The listing builds one solid part. Answer for the finished solid, in the listing's coordinates (mm). A direction names the side the tool comes from. Give positions to 0.01 mm unless a question says otherwise; leave off trailing zeros. Order: outer loops, then holes, each group sorted by start corner. A loop starts at its lowest first (then second) coordinate and runs counter-clockwise, first axis right, second up. Notation, with made-up numbers: M -33,9 L 16,9 A20 cw 16,22 Z; hole C 41,-13.5 d7. An arc over 180 degrees is marked long. Answer as a JSON object with one key per item and string values. Group by question number.
```python
from build123d import *

# Parameters (mm, degrees)
SKETCH1_R                          = 38.1
BOSS_EXTRUDE1_DEPTH                = 6.35
SKETCH2_R                          = 25.273
BOSS_EXTRUDE2_DEPTH                = 6.35
F_11_0_191_DIAMETER_HOLE1_D        = 4.8514
CIRPATTERN1_COUNT                  = 6
F_9_16_18_TAPPED_HOLE1_D           = 13.09624
F_9_16_18_TAPPED_HOLE1_CSINK_D     = 16.51
F_9_16_18_TAPPED_HOLE1_CSINK_ANGLE = 90
F_0_257_DIAMETER_HOLE1_D           = 6.5278


with BuildPart() as part:
    # Sketch1 → Boss-Extrude1 (new body)
    with BuildSketch(Plane(origin=(0, 0, 0), x_dir=(1, 0, 0), z_dir=(0, 1, 0))):
        with Locations(Location((0, 0, 0), (0, 0, 270))):
            Circle(SKETCH1_R)
    extrude(amount=BOSS_EXTRUDE1_DEPTH)

    # Sketch2 → Boss-Extrude2 (add)
    with BuildSketch(Plane(origin=(0, 0, 0), x_dir=(-1, 0, 0), z_dir=(0, -1, 0))):
        with Locations(Location((0, 0, 0), (0, 0, 270))):
            Circle(SKETCH2_R)
    extrude(amount=BOSS_EXTRUDE2_DEPTH)

    # #11 (0.191) Diameter Hole1 (through all)
    with Locations(Plane(origin=(0, 6.35, 0), x_dir=(1, 0, 0), z_dir=(0, 1, 0))):
        with Locations((0, 34.036)):
            f_11_0_191_diameter_hole1 = Hole(F_11_0_191_DIAMETER_HOLE1_D / 2)

    # CirPattern1: #11 (0.191) Diameter Hole1 ×6 about axis
    cirpattern1_axis = Axis((0, 0, 0), (0, 1, 0))
    for i in range(1, CIRPATTERN1_COUNT):
        add(f_11_0_191_diameter_hole1.rotate(cirpattern1_axis, i * 360 / CIRPATTERN1_COUNT), mode=Mode.SUBTRACT)

    # 9/16-18 Tapped Hole1 (through all)
    with Locations(Plane(origin=(0, 6.35, 0), x_dir=(1, 0, 0), z_dir=(0, 1, 0))):
        with Locations((0, 0)):
            CounterSinkHole(F_9_16_18_TAPPED_HOLE1_D / 2, F_9_16_18_TAPPED_HOLE1_CSINK_D / 2, counter_sink_angle=F_9_16_18_TAPPED_HOLE1_CSINK_ANGLE)

    # F (0.257) Diameter Hole1 (through all)
    with Locations(Plane(origin=(0, 6.35, 0), x_dir=(1, 0, 0), z_dir=(0, 1, 0))):
        with Locations((20.066, 0)):
            Hole(F_0_257_DIAMETER_HOLE1_D / 2)


solid = part.part
```
Item 1: Section C-C (y = 2.25) is taken. Count the separate pieces of the cut face and the enclosed holes in it, and give its area (3 significant figures).
Item 2: Section A-A (z = 0) is taken. Determine the outline of the cut face in (x, y) (3 decimals), and give its area (3 significant figures).
Item 3: Determine the mould class of faces 3 (the cylindrical face through (-27.235, 3.131, -17.947)), 4 (the cylindrical face through (9.68, -3.131, 23.346)), 5 (the flat face through (5, -6.35, 5)) for opening direction X: released by +X, released by -X, zero draft, split by the parting line, or undercut.
Item 4: Section D-D (x = -13) is taken. Determine the outline of the cut face in (y, z).
Item 5: Flat-ended cylindrical pins translate along their axes: P1, Ø3, axis at y = 3, z = 22.5, coming from the +X side; P2, Ø6.5, axis at x = -29.48, z = -17.02, coming from the -Y side; P3, Ø4, axis at y = -0.5, z = 16.5, coming from the +X side. Find the tip coordinate at first contact, or state that the pin passes through.
Item 6: A tool of negligible diameter and unlimited length cuts with its end or side. For faces 1 (the flat face through (-25, 0, 8)), 2 (the cylindrical face through (0.32, 3.13, -36.44)), from which of +Z, -Z, +X, -X, +Y, -Y can it reach the whole face along a straight path? Write none if from no direction.
Item 7: Consider probe 1 along Z at (x, y) = (-0.5, -4.5); probe 2 along X at (y, z) = (-2.5, -2); probe 3 along Y at (x, z) = (-14, 22.5). Determine where each line is inside the solid, lowest interval first. Write a range as from..to.
Item 8: Section B-B (x = 19.5) is taken. Determine the outline of the cut face in (y, z).
Values found:
{
 "1": {"separate pieces": "1", "enclosed holes": "8", "area": "4,280 mm^2"},
 "2": {"outline": "M -38.1,0 L -25.273,0 L -25.273,-6.35 L -6.548,-6.35 L -6.548,4.643 L -8.255,6.35 L -38.1,6.35 Z; M 6.548,-6.35 L 16.802,-6.35 L 16.802,6.35 L 8.255,6.35 L 6.548,4.643 Z; M 23.33,-6.35 L 25.273,-6.35 L 25.273,0 L 38.1,0 L 38.1,6.35 L 23.33,6.35 Z", "area": "553 mm^2"},
 "3": {"face 3": "undercut", "face 4": "split by the parting line", "face 5": "zero draft"},
 "4": {"outline": "M -6.35,-21.67 L 0,-21.67 L 0,-35.81 L 6.35,-35.81 L 6.35,35.81 L 0,35.81 L 0,21.67 L -6.35,21.67 Z"},
 "5": {"P1": "stops at x = 31.79", "P2": "stops at y = 0", "P3": "stops at x = 35.21"},
 "6": {"face 1": "-Y", "face 2": "+Y, -Y"},
 "7": {"probe 1": "z = -25.27..-6.53, 6.53..25.27", "probe 2": "x = -25.19..-6.24, 6.24..17.49, 22.65..25.19", "probe 3": "y = 0..6.35"},
 "8": {"outline": "M -6.35,-16.08 L 0,-16.08 L 0,-32.73 L 6.35,-32.73 L 6.35,-3.21 L -6.35,-3.21 Z; M -6.35,3.21 L 6.35,3.21 L 6.35,32.73 L 0,32.73 L 0,16.08 L -6.35,16.08 Z"}
}
